Design review of the part built by this model. Coordinates are the model's own, in mm. A direction names the side the tool comes from. Give positions to 0.01 mm unless a question says otherwise; leave off trailing zeros. Order: outer loops, then holes, each group sorted by start corner. A loop starts at its lowest first (then second) coordinate and runs counter-clockwise, first axis right, second up. Notation, with made-up numbers: M 52,59.25 L 106,59.25 A13 cw 106,80.25 Z; hole C 5.5,70 d10. An arc over 180 degrees is marked long. Answer as a JSON object with one key per item and string values.
from build123d import *

# Parameters (mm, degrees)
F0_R      = 13.5
F0_R_2    = 10.75
F1_DEPTH  = 5
F2_R      = 25
F2_R_2    = 13.5
F2_R_3    = 10.75
F3_DEPTH  = 7
F4_R      = 17.5
F5_DEPTH  = 27
F6_R      = 30
F6_R_2    = 17.5
F7_DEPTH  = 11
F8_R      = 22.5
F9_DEPTH  = 49
F10_R     = 15
F11_DEPTH = 4
F12_R     = 17
F12_R_2   = 15
F13_DEPTH = 5
F14_R     = 11.5
F15_DEPTH = 37
F16_R     = 10.75
F17_DEPTH = 103.001
F18_SIZE  = 0.5
F19_SIZE2 = 2.99999
F19_SIZE  = 7.49999
F20_SIZE  = 0.5
F22_R     = 11.5
F23_DEPTH = 1.1


# Not quite as in the source:
# - a fillet or chamfer is up to 0.001 mm smaller than in the source, because OpenCascade refuses the exact size


with BuildPart() as f1:
    # F0 (on Top) → F1 (new body)
    with BuildSketch(Plane.XY):
        Circle(F0_R)
        Circle(F0_R_2, mode=Mode.SUBTRACT)
    extrude(amount=F1_DEPTH)

    # F2 (on face) → F3 (join)
    with BuildSketch(Plane(origin=(0, 0, 0), x_dir=(1, 0, 0), z_dir=(0, 0, -1))):
        Circle(F2_R)
        Circle(F2_R_2, mode=Mode.SUBTRACT)
        Circle(F2_R_2)
        Circle(F2_R_3, mode=Mode.SUBTRACT)
    extrude(amount=F3_DEPTH)

    # F4 (on face) → F5 (join)
    with BuildSketch(Plane(origin=(0, 0, -7), x_dir=(1, 0, 0), z_dir=(0, 0, -1))):
        Circle(F4_R)
    extrude(amount=F5_DEPTH)

    # F6 (on face) → F7 (join)
    with BuildSketch(Plane(origin=(0, 0, -34), x_dir=(1, 0, 0), z_dir=(0, 0, -1))):
        Circle(F6_R)
        Circle(F6_R_2, mode=Mode.SUBTRACT)
        Circle(F6_R_2)
    extrude(amount=F7_DEPTH)

    # F8 (on face) → F9 (join)
    with BuildSketch(Plane(origin=(0, 0, -45), x_dir=(1, 0, 0), z_dir=(0, 0, -1))):
        Circle(F8_R)
    extrude(amount=F9_DEPTH)

    # F10 (on face) → F11 (join)
    with BuildSketch(Plane(origin=(0, 0, -94), x_dir=(1, 0, 0), z_dir=(0, 0, -1))):
        Circle(F10_R)
    extrude(amount=F11_DEPTH)

    # F12 (on face) → F13 (join)
    with BuildSketch(Plane(origin=(0, 0, -98), x_dir=(1, 0, 0), z_dir=(0, 0, -1))):
        Circle(F12_R)
        Circle(F12_R_2, mode=Mode.SUBTRACT)
        Circle(F12_R_2)
    extrude(amount=F13_DEPTH)

    # F14 (on face) → F15 (cut)
    with BuildSketch(Plane(origin=(0, 0, -103), x_dir=(1, 0, 0), z_dir=(0, 0, -1))):
        Circle(F14_R)
    extrude(amount=-F15_DEPTH, mode=Mode.SUBTRACT)

    # F16 (on face) → F17 (cut, through all)
    with BuildSketch(Plane.XY):
        Circle(F16_R)
    extrude(amount=-F17_DEPTH, mode=Mode.SUBTRACT)

    # F18
    f18_edges = [f1.edges().sort_by_distance(p)[0] for p in [
        (-11.5, 0, -103),
        (-22.5, 0, -94),
        (-30, 0, -45),
        (-30, 0, -34),
        (-25, 0, 0),
        (-13.5, 0, 5),
        (-10.75, 0, 5),
    ]]
    chamfer(f18_edges, length=F18_SIZE)

    # F19 (size 7.5 and 3 in the source; OpenCascade refuses exactly that, so slightly less here)
    f19_edges = [f1.edges().sort_by_distance(p)[0] for p in [
        (-25, 0, -7),
    ]]
    f19_side = f1.faces().sort_by_distance((-24.292893, 0, -7))[0]
    chamfer(f19_edges, length=F19_SIZE, length2=F19_SIZE2, reference=f19_side)

    # F20
    f20_edges = [f1.edges().sort_by_distance(p)[0] for p in [
        (-25, 0, -4.00001),
    ]]
    chamfer(f20_edges, length=F20_SIZE)

    # F22 (on offset) → F23 (cut)
    with BuildSketch(Plane.XY.offset(1)):
        Circle(F22_R)
    extrude(amount=-F23_DEPTH, mode=Mode.SUBTRACT)


solid = f1.part
(1) We need section B-B (z = -15.5). Write out the cut boundary in (x, y).
Checked values:
{"outline": "C 0,0 d35; hole C 0,0 d21.5"}
(2) To check wall thickness, follow L1, parallel to Y at x = 0, z = 2.7; L2, parallel to X at y = 0, z = -80.5; L3, parallel to Y at x = 0, z = -15. State the ranges of each line that lie inside material, in increasing order. Write a range as from..to.
Checked values:
{"L1": "y = -13.5..-10.75, 10.75..13.5", "L2": "x = -22.5..-11.5, 11.5..22.5", "L3": "y = -17.5..-10.75, 10.75..17.5"}
(3) We need section A-A (z = -37.5). Write out the cut boundary in (x, y).
Checked values:
{"outline": "C 0,0 d60; hole C 0,0 d21.5"}
(4) Insertion check: pin 1 (2 mm diameter, centred on y = -18.5, z = -53, fed in from -X); pin 2 (5 mm diameter, centred on y = 2.5, z = -88.5, fed in from +X); pin 3 (8 mm diameter, centred on y = -17, z = -66, fed in from -X). Each pin has a flat end and moves straight along its axis. Give the tip position at first contact, or say it passes through.
Checked values:
{"pin 1": "stops at x = -14.14", "pin 2": "stops at x = 22.5", "pin 3": "stops at x = -18.36"}
(5) Draft analysis for pull direction Y (two halves, no side actions). For faces 1 (the cylindrical face through (-1.5, -11.4, -84.5)), 2 (the flat face through (-6, 10, 5)), 3 (the cylindrical face through (-14.985, -0.66, -95.972)), state which applies: +Y half, -Y half, draft (parallel to the pull), parting line (faces both ways), or undercut.
Checked values:
{"face 1": "undercut", "face 2": "draft", "face 3": "parting line"}
(6) Tool access review of faces 4 (the cylindrical face through (-1.4, 10.66, -32.59)), 5 (the cylindrical face through (-2.93, -13.18, 2.22)), 6 (the flat face through (13, 13, -34)), 7 (the flat face through (-7, 22, -45)), 8 (the flat face through (4, -12, -103)): name each direction out of +Z, -Z, +X, -X, +Y, -Y from which nothing blocks a thin tool from reaching the whole face with its end or side.
Checked values:
{"face 4": "+Z, -Z", "face 5": "+Z", "face 6": "none", "face 7": "-Z", "face 8": "-Z, +X, -X, +Y, -Y"}
